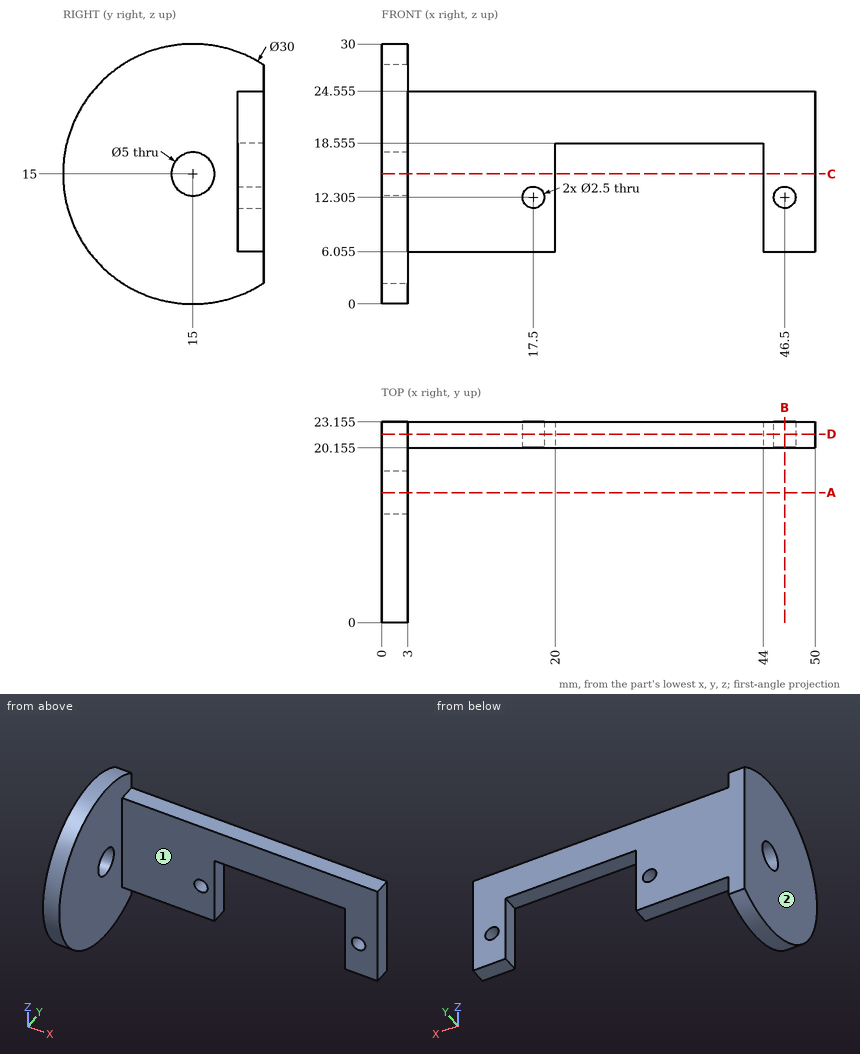
Answer from the drawing. Dimensions are ordinates in mm from the lowest x, y and z of the part. A direction names the side the tool comes from. Give positions to 0.01 mm unless a question says otherwise; leave off trailing zeros. Loops run counter-clockwise (first coordinate to the right, second up) from the corner with the lowest first, then second, coordinate; pieces in that order, holes last. Notation, with made-up numbers: (22, 19) -> (70, 19) arc R19 cw to (70, 55) -> close; hole circle Ø3 at (76.5, 29). An arc over 180 degrees is marked (long way). Use a Markdown table: item, result.
Q1. Section A-A, the plane y = 15 is taken. Determine the outline of the cut face in (x, z).
Solved:
| item | result |
|---|---|
| outline | (0, 0) -> (3, 0) -> (3, 12.5) -> (0, 12.5) -> close; (0, 17.5) -> (3, 17.5) -> (3, 30) -> (0, 30) -> close |
Q2. Section D-D, the plane y = 21.75 is taken. Count the separate pieces of the cut face and the enclosed holes in it, then the cut area to 3 significant figures.
Solved:
| item | result |
|---|---|
| separate pieces | 1 |
| enclosed holes | 2 |
| area | 640 mm^2 |
Q3. Section B-B, the plane x = 46.5 is taken. Determine the outline of the cut face in (y, z) (1 decimal), then the cut area to 3 significant figures.
Solved:
| item | result |
|---|---|
| outline | (20.2, 6.1) -> (23.2, 6.1) -> (23.2, 11.1) -> (20.2, 11.1) -> close; (20.2, 13.6) -> (23.2, 13.6) -> (23.2, 24.6) -> (20.2, 24.6) -> close |
| area | 48.0 mm^2 |
Q4. Find the intervals of material crossed by line 1 along Z through (x, y) = (2.05, 15); line 2 along Z through (x, y) = (46.5, 20.85) (1 decimal); line 3 along X through (y, z) = (20.75, 11.75), in increasing order.
Solved:
| item | result |
|---|---|
| line 1 | z = 0 to 12.5, 17.5 to 30 |
| line 2 | z = 6.1 to 11.1, 13.6 to 24.6 |
| line 3 | x = 0 to 16.38, 18.62 to 20, 44 to 45.38, 47.62 to 50 |
Q5. Each of these flat-tipped pins is pushed along its axis until it touches: pin 1 (3 mm diameter, centred on x = 17.5, z = 12.31, fed in from -Y) (1 decimal); pin 2 (0.9 mm diameter, centred on x = 47, y = 21.5, fed in from -Z) (1 decimal); pin 3 (0.9 mm diameter, centred on x = 34.5, y = 22.5, fed in from +Z) (1 decimal). Where does it stop, or does it pass through?
Solved:
| item | result |
|---|---|
| pin 1 | stops at y = 20.2 |
| pin 2 | stops at z = 6.1 |
| pin 3 | stops at z = 24.6 |
Q6. Section C-C, the plane z = 15 is taken. Determine the outline of the cut face in (x, y) (1 decimal).
Solved:
| item | result |
|---|---|
| outline | (0, 0) -> (3, 0) -> (3, 12.5) -> (0, 12.5) -> close; (0, 17.5) -> (3, 17.5) -> (3, 20.2) -> (20, 20.2) -> (20, 23.2) -> (0, 23.2) -> close; (44, 20.2) -> (50, 20.2) -> (50, 23.2) -> (44, 23.2) -> close |
Q7. A tool of negligible diameter and unlimited length cuts with its end or side. For the marked faces 1 and 2, from which of +Z, -Z, +X, -X, +Y, -Y can it reach the whole face along a straight path? Write none if from no direction.
Solved:
| item | result |
|---|---|
| face 1 | +Z, -Z, +X, -Y |
| face 2 | +Z, -Z, -X, +Y, -Y |
